```python
from build123d import *

# Parameters (mm, degrees)
BOSS_EXTRUDE1_DEPTH      = 14
BOSS_EXTRUDE1_DEPTH_BACK = 14
FILLET2_R                = 3.175
FILLET3_R                = 1.016
FILLET4_R                = 1.5875
SKETCH3_R                = 9.0297
CUT_EXTRUDE1_DEPTH       = 3.048


with BuildPart() as part:
    # Sketch1 → Boss-Extrude1 (new, two sides: drawn at the far end of the back side and taken through both)
    with BuildSketch(Plane(origin=(0, 0, 0), x_dir=(0, 0, -1), z_dir=(1, 0, 0)).offset(-BOSS_EXTRUDE1_DEPTH_BACK)):
        Polygon((-16.0655, -10.325348422), (-9.7155, -10.325348422), (-9.7155, -6.263815771), (-14.478, -5.424058525), (-14.478, 11.008), (0, 11.008), (14.478, 11.008), (14.478, -5.424058525), (9.7155, -6.263815771), (9.7155, -10.325348422), (16.0655, -10.325348422), (16.0655, 17.358), (0, 17.358), (-16.0655, 17.358), align=None)
    extrude(amount=BOSS_EXTRUDE1_DEPTH + BOSS_EXTRUDE1_DEPTH_BACK)

    # Fillet2
    fillet2_edges = [part.edges().sort_by_distance(p)[0] for p in [
        (0, -10.325348422, 16.0655),
        (0, -10.325348422, -16.0655),
    ]]
    fillet(fillet2_edges, radius=FILLET2_R)

    # Fillet3
    fillet3_edges = [part.edges().sort_by_distance(p)[0] for p in [
        (0, -5.424058525, -14.478),
        (0, 11.008, -14.478),
        (0, 11.008, 14.478),
        (0, -5.424058525, 14.478),
    ]]
    fillet(fillet3_edges, radius=FILLET3_R)

    # Fillet4
    fillet4_edges = [part.edges().sort_by_distance(p)[0] for p in [
        (0, -6.263815771, 9.7155),
        (0, -10.325348422, 9.7155),
        (0, -10.325348422, -9.7155),
        (0, -6.263815771, -9.7155),
    ]]
    fillet(fillet4_edges, radius=FILLET4_R)

    # Sketch3 → Cut-Extrude1 (cut)
    with BuildSketch(Plane(origin=(0, 11.008, 0), x_dir=(-1, 0, 0), z_dir=(0, -1, 0))):
        with Locations(Location((0, 0, 0), (0, 0, 90))):
            Circle(SKETCH3_R)
    extrude(amount=-CUT_EXTRUDE1_DEPTH, mode=Mode.SUBTRACT)


solid = part.part
```
Part model, mm, in its own coordinate system. A direction names the side the tool comes from. Give positions to 0.01 mm unless a question says otherwise; leave off trailing zeros. Order: outer loops, then holes, each group sorted by start corner. A loop starts at its lowest first (then second) coordinate and runs counter-clockwise, first axis right, second up. Notation, with made-up numbers: M 0.5,36.5 L 50.5,36.5 A19 cw 50.5,73.5 Z; hole C 64,81 d10. An arc over 180 degrees is marked long. Use a Markdown table: item, result. Add a question column.
(1) Drop flat-ended pins along their axis: P1, Ø1, axis at x = 8, z = -8.5, coming from the -Y side; P2, Ø5, axis at x = -2.5, z = -7.5, coming from the -Y side; P3, Ø4, axis at x = 0, z = 8.5, coming from the -Y side. Give the stop position or say it passes through.
(2) Mould opens along Z. For faces 1 (the face through (0, -10.325, 12)), 2 (the face through (-0.196, -5.806, 12.315)), 3 (the face through (0.2, -9.42, -15.11)), 4 (the face through (0, 3, 14.478)) say: +Z half, -Z half, draft (parallel to the pull), parting line (faces both ways), or undercut.
(3) 3-axis set-ups, long thin cutter, end or side, ignore diameter. For faces 5 (the face through (0, -8, 9.716)), 6 (the face through (14, 12, -1)), 7 (the face through (0, 14.056, 0)), 8 (the face through (0, 5, -16.066)), 9 (the face through (0.2, 10.7, 14.19)): which of +Z, -Z, +X, -X, +Y, -Y reach the whole face in a straight line?
(4) Saw through at A-A, the plane y = 7.75. Give the cut face in (x, z), and give its area (3 significant figures).
(5) Saw through at B-B, the plane z = 0. Give the cut face in (x, y).
(6) Probe line 1 along X through (y, z) = (11.8, 0); line 2 along Z through (x, y) = (11.75, 5.75); line 3 along Y through (x, z) = (-7.5, -10). List the from-to ranges inside material, lowest first. Write a range as [from, to].
Answer key:
| question | item | result |
|---|---|---|
| 1 | P1 | y = 11.01 |
| 1 | P2 | y = -9.64 |
| 1 | P3 | y = -10.11 |
| 2 | face 1 | draft |
| 2 | face 2 | undercut |
| 2 | face 3 | -Z half |
| 2 | face 4 | undercut |
| 3 | face 5 | +X, -X, -Y |
| 3 | face 6 | +Z, -Z, +X, +Y, -Y |
| 3 | face 7 | -Y |
| 3 | face 8 | -Z, +X, -X, +Y, -Y |
| 3 | face 9 | +X, -X |
| 4 | outline | M -14,-16.07 L 14,-16.07 L 14,-14.48 L -14,-14.48 Z; M -14,14.48 L 14,14.48 L 14,16.07 L -14,16.07 Z |
| 4 | area | 88.9 mm^2 |
| 5 | outline | M -14,11.01 L -9.03,11.01 L -9.03,14.06 L 9.03,14.06 L 9.03,11.01 L 14,11.01 L 14,17.36 L -14,17.36 Z |
| 6 | line 1 | [-14, -9.03], [9.03, 14] |
| 6 | line 2 | [-16.07, -14.48], [14.48, 16.07] |
| 6 | line 3 | [-9.64, -6.69], [11.01, 17.36] |
